Input: dimensioned drawing with shaded views. Units: mm. Origin: part minimum x, y, z. A direction names the side the tool comes from. Round coordinates to 2 decimals unless told otherwise and drop trailing zeros. Loops run counter-clockwise (first coordinate to the right, second up) from the corner with the lowest first, then second, coordinate; pieces in that order, holes last. Notation, with made-up numbers: (12, 70) -> (44, 70) arc R15 cw to (44, 88) -> close; hole circle Ø2 at (69, 24). An arc over 180 degrees is marked (long way). Answer as a JSON object with one key per item and string values.
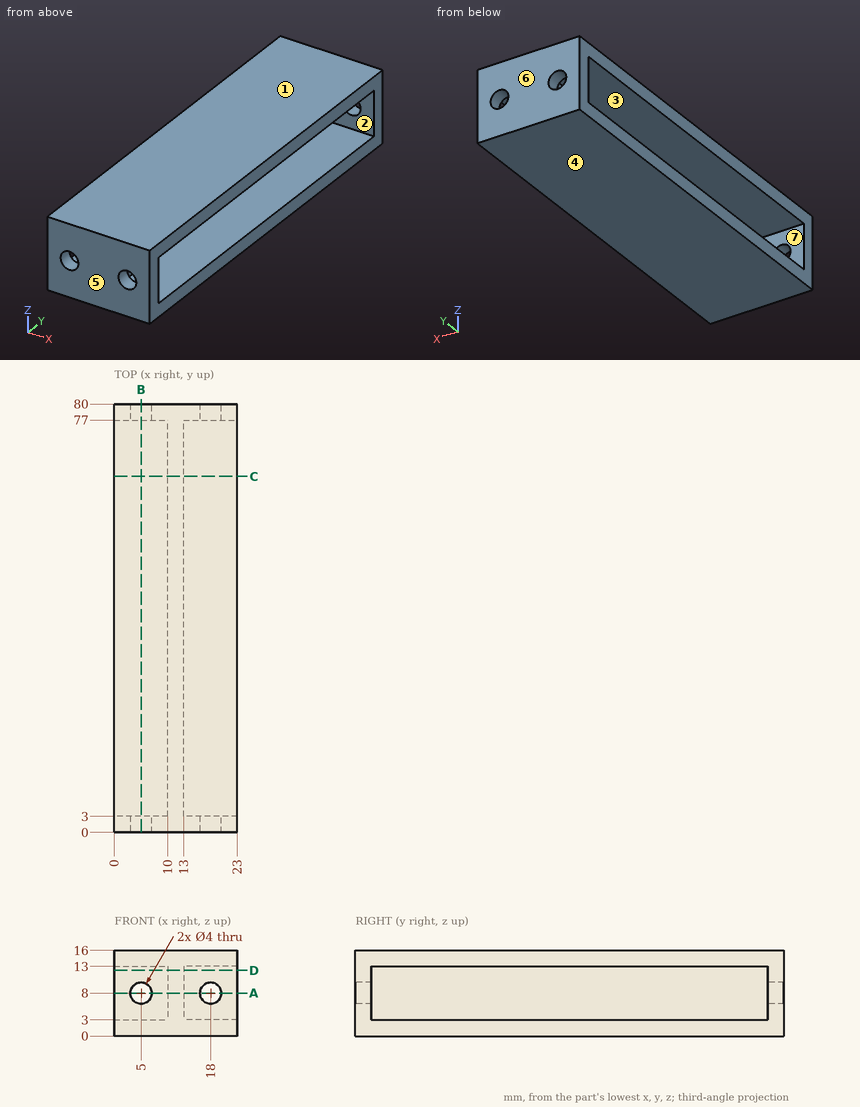
1) Draft query along Y for the marked faces 4, 5, 6 and 7. Return one class per face: +Y half, -Y half, draft (parallel to the pull), parting line (faces both ways), or undercut.
Output:
{"face 4": "draft", "face 5": "-Y half", "face 6": "+Y half", "face 7": "undercut"}
2) Reachability of the marked faces 1, 2 and 3 from +Z, -Z, +X, -X, +Y, -Y: full face, straight path, thin tool, end or side. Return the list, or none.
Output:
{"face 1": "+Z, +X, -X, +Y, -Y", "face 2": "+X", "face 3": "-X"}
3) Contact query for flat-ended pins moving along their axis: P1, Ø4, axis at x = 14, y = 12, coming from the -Z side; P2, Ø2.5, axis at x = 18, z = 8, coming from the +Y side; P3, Ø2, axis at y = 62.5, z = 5.5, coming from the +X side; P4, Ø1.5, axis at y = 58.5, z = 6, coming from the -X side. Output: stop coordinate, or through.
Output:
{"P1": "stops at z = 0", "P2": "passes through", "P3": "stops at x = 13", "P4": "stops at x = 10"}
4) Section B-B, the plane x = 5. Output: boundary loops of the cut face in (y, z), plus the area to 3 significant figures.
Output:
{"outline": "(0, 0) -> (80, 0) -> (80, 6) -> (77, 6) -> (77, 3) -> (3, 3) -> (3, 6) -> (0, 6) -> close; (0, 10) -> (3, 10) -> (3, 13) -> (77, 13) -> (77, 10) -> (80, 10) -> (80, 16) -> (0, 16) -> close", "area": "516 mm^2"}
5) Section C-C, the plane y = 66.5. Output: boundary loops of the cut face in (x, z).
Output:
{"outline": "(0, 0) -> (23, 0) -> (23, 3) -> (13, 3) -> (13, 13) -> (23, 13) -> (23, 16) -> (0, 16) -> (0, 13) -> (10, 13) -> (10, 3) -> (0, 3) -> close"}
6) Section A-A, the plane z = 8. Output: boundary loops of the cut face in (x, y).
Output:
{"outline": "(0, 0) -> (3, 0) -> (3, 3) -> (0, 3) -> close; (0, 77) -> (3, 77) -> (3, 80) -> (0, 80) -> close; (7, 0) -> (16, 0) -> (16, 3) -> (13, 3) -> (13, 77) -> (16, 77) -> (16, 80) -> (7, 80) -> (7, 77) -> (10, 77) -> (10, 3) -> (7, 3) -> close; (20, 0) -> (23, 0) -> (23, 3) -> (20, 3) -> close; (20, 77) -> (23, 77) -> (23, 80) -> (20, 80) -> close"}
7) Section D-D, the plane z = 12.25. Output: boundary loops of the cut face in (x, y).
Output:
{"outline": "(0, 0) -> (23, 0) -> (23, 3) -> (13, 3) -> (13, 77) -> (23, 77) -> (23, 80) -> (0, 80) -> (0, 77) -> (10, 77) -> (10, 3) -> (0, 3) -> close"}
8) Ray query, probe 1 along X at (y, z) = (1.6, 8); probe 2 along Z at (x, y) = (6.25, 41); probe 3 along Z at (x, y) = (18, 0.9). Return the intervals inside material, ascending.
Output:
{"probe 1": "x = 0 to 3, 7 to 16, 20 to 23", "probe 2": "z = 0 to 3, 13 to 16", "probe 3": "z = 0 to 6, 10 to 16"}
